```python
from build123d import *

# Parameters (mm, degrees)
EXTRUDE_4_DEPTH     = 80
CUT_EXTRUDE_1_DEPTH = 80
FILLET_3_R          = 2
FILLET_4_R          = 2
CUT_EXTRUDE_2_DEPTH = 90
CUT_EXTRUDE_3_DEPTH = 90
FILLET_5_R          = 2
FILLET_6_R          = 2


with BuildPart() as part:
    # 草图1 → 凸台-拉伸4 (new body)
    with BuildSketch(Plane(origin=(0, 0, 0), x_dir=(1, 0, 0), z_dir=(0, 1, 0))):
        with BuildLine():
            Line((-58.430824656, -54.95766375), (91.569175344, -54.95766375))
            ThreePointArc((91.569175344, -54.95766375), (16.569175344, -21.101446527), (-58.430824656, -54.95766375))
        make_face()
    extrude(amount=EXTRUDE_4_DEPTH)

    # 草图6 → 切除-拉伸1 (cut)
    with BuildSketch(Plane(origin=(0, 80, 0), x_dir=(1, 0, 0), z_dir=(0, 1, 0))):
        with BuildLine():
            Line((16.569175344, -54.95766375), (-53.430824656, -54.95766375))
            Line((-53.430824656, -54.95766375), (-44.284141383, -47.292975133))
            ThreePointArc((-44.284141383, -47.292975133), (-41.278424436, -45.559608468), (-37.861326704, -44.95766375))
            Line((-37.861326704, -44.95766375), (16.569175344, -44.95766375))
            Line((16.569175344, -44.95766375), (70.999677391, -44.95766375))
            ThreePointArc((70.999677391, -44.95766375), (74.416775124, -45.559608468), (77.422492071, -47.292975133))
            Line((77.422492071, -47.292975133), (86.569175344, -54.95766375))
            Line((86.569175344, -54.95766375), (16.569175344, -54.95766375))
        make_face()
    extrude(amount=-CUT_EXTRUDE_1_DEPTH, mode=Mode.SUBTRACT)

    # 圆角3
    fillet_3_edges = [part.edges().sort_by_distance(p)[0] for p in [
        (-58.430824656, 40, 54.95766375),
    ]]
    fillet(fillet_3_edges, radius=FILLET_3_R)

    # 圆角4
    fillet_4_edges = [part.edges().sort_by_distance(p)[0] for p in [
        (91.569175344, 40, 54.95766375),
    ]]
    fillet(fillet_4_edges, radius=FILLET_4_R)

    # 草图7 → 切除-拉伸2 (cut, symmetric)
    with BuildSketch(Plane(origin=(0, 0, 0), x_dir=(0, 0, -1), z_dir=(1, 0, 0))):
        Polygon((-34.95766375, 20), (-21.101446527, 20), (-21.101446527, 60), (-34.95766375, 60), (-34.95766375, 40), align=None)
    extrude(amount=CUT_EXTRUDE_2_DEPTH, both=True, mode=Mode.SUBTRACT)

    # 草图8 → 切除-拉伸3 (cut, symmetric)
    with BuildSketch(Plane(origin=(0, 0, 0), x_dir=(0, 0, -1), z_dir=(1, 0, 0))):
        Polygon((-46.566974306, 40), (-46.566974306, 20), (-51.566974306, 20), (-51.566974306, 40), (-51.566974306, 60), (-46.566974306, 60), align=None)
    extrude(amount=CUT_EXTRUDE_3_DEPTH, both=True, mode=Mode.SUBTRACT)

    # 圆角5
    # the kernel refuses this fillet: 2 mm, written as the material it takes off along each edge
    with BuildSketch(Plane(origin=(-49.384533414, 20, 51.566974306), x_dir=(-0.7664688616948695, 0, 0.6422814679345583), z_dir=(0, 1, 0))) as fillet_5_piece_1:
        with BuildLine():
            CenterArc((FILLET_5_R * 2.75030333255, -FILLET_5_R), FILLET_5_R, 90, 140.037846047)
            Line((FILLET_5_R * 2.10802186461, -FILLET_5_R * 1.76646886169), (0, 0))
            Line((0, 0), (FILLET_5_R * 2.75030333255, 0))
        make_face()
    extrude(amount=40, mode=Mode.SUBTRACT)

    # 圆角6
    # the kernel refuses this fillet: 2 mm, written as the material it takes off along each edge
    with BuildSketch(Plane(origin=(82.522884101, 60, 51.566974306), x_dir=(1, 0, 0), z_dir=(0, -1, 0))) as fillet_6_piece_1:
        with BuildLine():
            CenterArc((FILLET_6_R * 2.75030333255, FILLET_6_R), FILLET_6_R, 129.962153953, 140.037846047)
            Line((FILLET_6_R * 2.10802186461, FILLET_6_R * 1.76646886169), (0, 0))
            Line((0, 0), (FILLET_6_R * 2.75030333255, 0))
        make_face()
    extrude(amount=40, mode=Mode.SUBTRACT)


solid = part.part
```
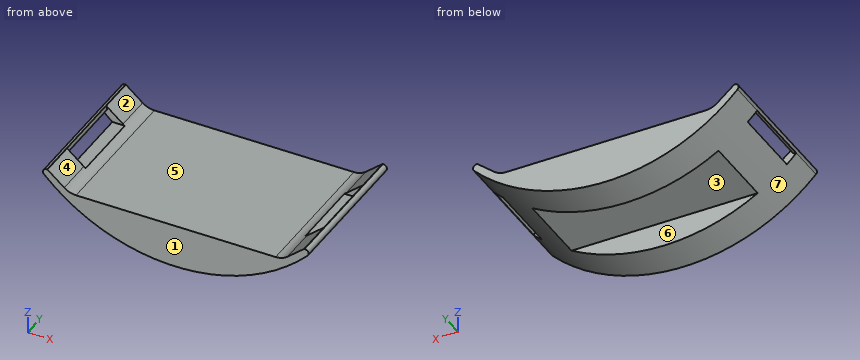
CAD build for the part. Positions are in the model's coordinates, mm. Face numbers are marked on the shaded views. A direction names the side the tool comes from. Coordinates: 2 decimals unless noted, no trailing zeros. Write each loop counter-clockwise with the first axis right and the second up, starting at its lowest first coordinate (ties: lowest second). Pieces come first, ordered by that corner, then holes. Notation, with made-up numbers: (58, 39.25) -> (69, 39.25) arc R24 cw to (69, 53.25) -> close; hole circle Ø2 at (-18, 78.5). An arc over 180 degrees is marked (long way). Return JSON: item names as keys, results as strings. Group by question number.
Q1. Cut at A-A, the plane z = 28.5. Give the cut face in (x, y).
Q2. Which spindle directions (+Z, -Z, +X, -X, +Y, -Y) get a long thin tool onto all of the face, cutting with end or side? Do the marked faces 1, 2 and 3. Say none if no direction does.
Q3. Drill centre lines: line 1 (Z direction, x = 36.5, y = 21.5); line 2 (X direction, y = 50.5, z = 52.5); line 3 (X direction, y = 36, z = 53.5). Where is each one in solid material? Low to high.
Q4. Cut at C-C, the plane x = 21. Give the cut face in (y, z).
Q5. Pull direction X, two halves, no side cores. Call the marked faces 4, 5, 6 and 7: released by +X, released by -X, zero draft, split by the parting line, or undercut.
Q6. Flat gauge pins, fed straight in: pin 1 (10 mm diameter, centred on x = 22, y = 44, fed in from +Z); pin 2 (4 mm diameter, centred on x = -10.5, y = 18, fed in from -Z); pin 3 (10 mm diameter, centred on y = 64, z = 38.5, fed in from +X). Where does each tip first touch, or does it go through?
Q7. Cut at D-D, the plane y = 52. Give the cut face in (x, z).
Q8. Cut at B-B, the plane y = 15. Give the cut face in (x, z).
Returned:
{
 "1": {"outline": "(-21.18, 0) -> (54.32, 0) -> (54.32, 20) -> (-21.18, 20) -> close; (-21.18, 60) -> (54.32, 60) -> (54.32, 80) -> (-21.18, 80) -> close"},
 "2": {"face 1": "+Z, -Z, +X, -X, -Y", "face 2": "+Z, +Y, -Y", "face 3": "-Z, +X, -X"},
 "3": {"line 1": "z = 34.96 to 44.96", "line 2": "x = -55.81 to -53.19, 86.33 to 88.95", "line 3": "x = -55.79 to -52.89, 86.02 to 88.92"},
 "4": {"outline": "(0, 21.2) -> (20, 21.2) -> (20, 34.96) -> (60, 34.96) -> (60, 21.2) -> (80, 21.2) -> (80, 44.96) -> (0, 44.96) -> close"},
 "5": {"face 4": "undercut", "face 5": "undercut", "face 6": "zero draft", "face 7": "split by the parting line"},
 "6": {"pin 1": "stops at z = 44.96", "pin 2": "stops at z = 24.29", "pin 3": "stops at x = 79.64"},
 "7": {"outline": "(-55.3, 51.57) -> (-54.89, 51.57) arc R2 ccw to (-53.45, 54.96) -> (-53.86, 54.96) arc R2 ccw to start; (-50.1, 46.57) arc R100 ccw to (-34.22, 34.96) -> (67.36, 34.96) arc R100 ccw to (83.24, 46.57) -> (76.44, 46.57) arc R10 cw to (71, 44.96) -> (-37.86, 44.96) arc R10 cw to (-43.3, 46.57) -> close; (86.59, 54.96) arc R2 ccw to (88.02, 51.57) -> (88.44, 51.57) arc R2 ccw to (87, 54.96) -> close"},
 "8": {"outline": "(-55.3, 51.57) arc R100 ccw to (88.44, 51.57) arc R2 ccw to (87, 54.96) -> (86.57, 54.96) -> (77.42, 47.29) arc R10 cw to (71, 44.96) -> (-37.86, 44.96) arc R10 cw to (-44.28, 47.29) -> (-53.43, 54.96) -> (-53.86, 54.96) arc R2 ccw to start"}
}
